Could you check a few things on this model? Use its own coordinates, in mm. Coordinates: 2 decimals unless noted, no trailing zeros. Loops run counter-clockwise (first coordinate to the right, second up) from the corner with the lowest first, then second, coordinate; pieces in that order, holes last. Notation, with made-up numbers: M 2,17.5 L 54,17.5 A27 ccw 54,50.5 Z; hole C -19.75,65 d8. An arc over 180 degrees is marked long. Return JSON: item names as keys, results as strings. Group by question number.
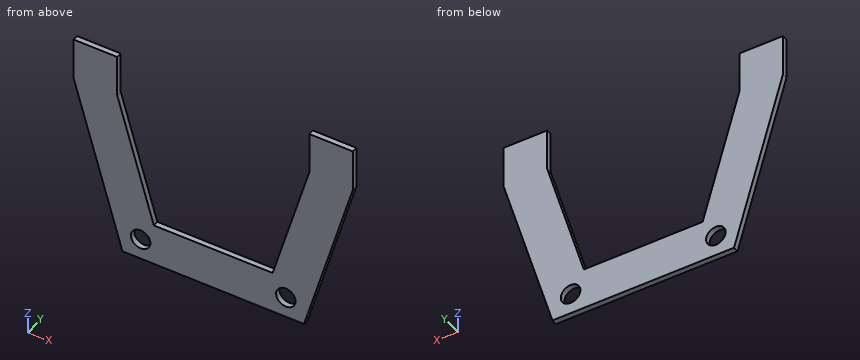
from build123d import *

# Parameters (mm, degrees)
F1_DEPTH = 2
F3_D     = 7


with BuildPart() as f1:
    # F0 (on Front) → F1 (new body)
    with BuildSketch(Plane.XZ):
        Polygon((-50, 22.5), (-32.5, -37.5), (32.5, -37.5), (50, 22.5), (50, 37.5), (34.375, 37.5), (34.375, 22.5), (21.25, -22.5), (-21.25, -22.5), (-34.375, 22.5), (-34.375, 37.5), (-50, 37.5), align=None)
    extrude(amount=F1_DEPTH)

    # F3 (through all)
    with Locations(Plane.XZ.offset(2)):
        with Locations((-26, -30), (26, -30)):
            Hole(F3_D / 2)


solid = f1.part
(1) Will these pins go through, and if not, where does the flat tip stop? P1, Ø12, axis at x = 27, z = 9.5, coming from the -Y side; P2, Ø5.5, axis at x = 26, z = -30, coming from the -Y side.
(2) If I drill on L1, parallel to X at y = -1.5, z = 31 (3 decimals); L2, parallel to X at y = -1.8, z = -31.5; L3, parallel to X at y = -0.8, z = -33, over which ranges is the centre line in solid material (lowest first)? Write a range as [from, to].
(3) Imagine slicing it at B-B, the plane x = -26. Write out the boundary of the cut face in (y, z).
(4) Imagine slicing it at D-D, the plane z = 13. Write out the boundary of the cut face in (x, y).
(5) Imagine slicing it at A-A, the plane y = -1.25. Write out the boundary of the cut face in (x, z) (3 decimals).
(6) Imagine slicing it at C-C, the plane z = -30. Write out the boundary of the cut face in (x, y), then the cut area to 3 significant figures.
Checks:
{
 "1": {"P1": "y = -2", "P2": "through"},
 "2": {"L1": "[-50, -34.375], [34.375, 50]", "L2": "[-34.25, -29.16], [-22.84, 22.84], [29.16, 34.25]", "L3": "[-33.81, -27.8], [-24.2, 24.2], [27.8, 33.81]"},
 "3": {"outline": "M -2,-37.5 L 0,-37.5 L 0,-33.5 L -2,-33.5 Z; M -2,-26.5 L 0,-26.5 L 0,-6.21 L -2,-6.21 Z"},
 "4": {"outline": "M -47.23,-2 L -31.6,-2 L -31.6,0 L -47.23,0 Z; M 31.6,-2 L 47.23,-2 L 47.23,0 L 31.6,0 Z"},
 "5": {"outline": "M -50,22.5 L -32.5,-37.5 L 32.5,-37.5 L 50,22.5 L 50,37.5 L 34.375,37.5 L 34.375,22.5 L 21.25,-22.5 L -21.25,-22.5 L -34.375,22.5 L -34.375,37.5 L -50,37.5 Z; hole C -26,-30 d7; hole C 26,-30 d7"},
 "6": {"outline": "M -34.69,-2 L -29.5,-2 L -29.5,0 L -34.69,0 Z; M -22.5,-2 L 22.5,-2 L 22.5,0 L -22.5,0 Z; M 29.5,-2 L 34.69,-2 L 34.69,0 L 29.5,0 Z", "area": "111 mm²"}
}
